Geometry: see drawing. Coordinates: mm, zero at the bounding-box minimum. A direction names the side the tool comes from. Coordinates: 2 decimals unless noted, no trailing zeros. Loops run counter-clockwise (first coordinate to the right, second up) from the corner with the lowest first, then second, coordinate; pieces in that order, holes last.
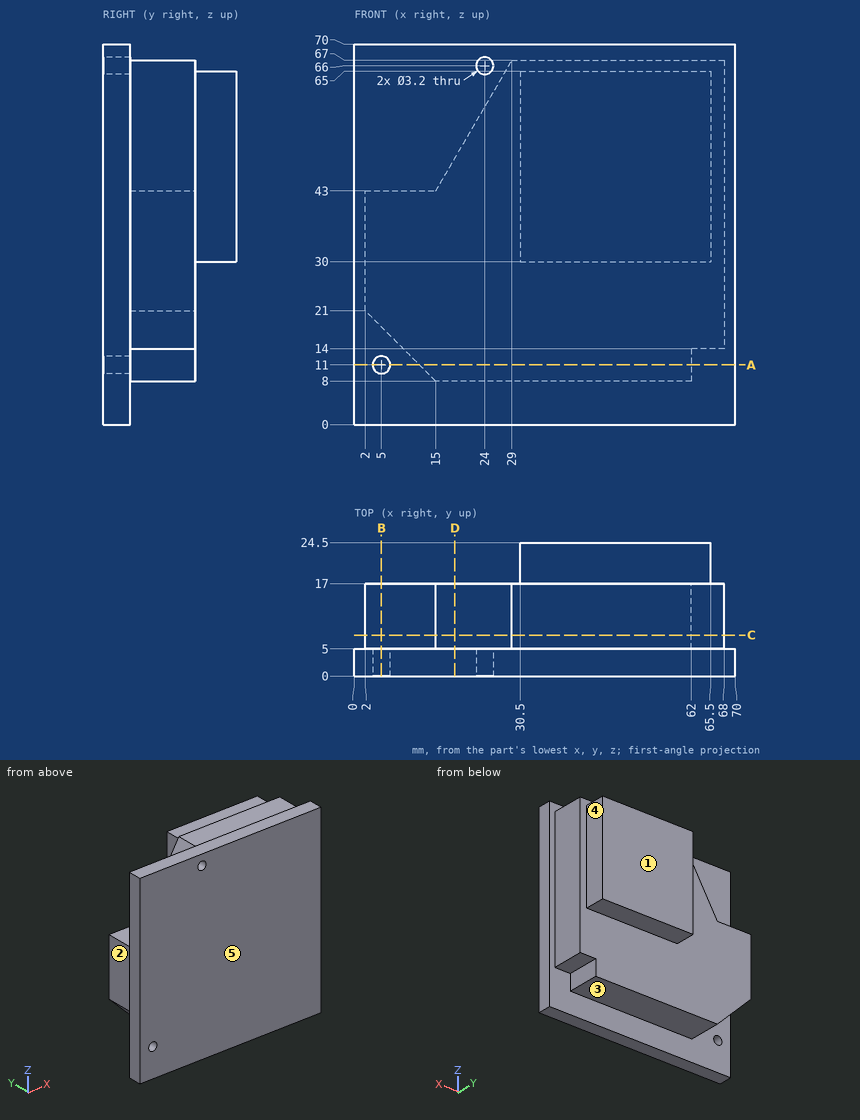
Item 1: Contact query for flat-ended pins moving along their axis: P1, Ø17.5, axis at x = 22.5, z = 31.5, coming from the +Y side; P2, Ø10, axis at x = 17, y = 20, coming from the +Z side; P3, Ø2.5, axis at x = 5, z = 11, coming from the -Y side; P4, Ø2, axis at x = 55.5, y = 18.5, coming from the -Z side. Output: stop coordinate, or through.
Result:
P1: stops at y = 24.5
P2: stops at z = 53.29
P3: passes through
P4: stops at z = 30
Item 2: Section query A-A (z = 11). Output: boundary loops of the cut face in (x, y).
Result:
outline: (0, 0) - (3.4, 0) - (3.4, 5) - (0, 5) - close; (6.6, 0) - (70, 0) - (70, 5) - (62, 5) - (62, 17) - (12, 17) - (12, 5) - (6.6, 5) - close
Item 3: Reachability of the marked faces 1, 2, 3, 4 and 5 from +Z, -Z, +X, -X, +Y, -Y: full face, straight path, thin tool, end or side. Return the list, or none.
Result:
face 1: +Z, -Z, +X, -X, +Y
face 2: +Z, -Z, -X, +Y
face 3: -Z, +X, -X, +Y
face 4: +Z, -Z, +X, +Y
face 5: +Z, -Z, +X, -X, -Y
Item 4: Section query C-C (y = 7.5). Output: boundary loops of the cut face in (x, z), then the cut area to 3 significant figures.
Result:
outline: (2, 21) - (15, 8) - (62, 8) - (62, 14) - (68, 14) - (68, 67) - (29, 67) - (15, 43) - (2, 43) - close
area: 3,290 mm2
Item 5: Line query: L1, parallel to Z at x = 5, y = 1.75; L2, parallel to Z at x = 24, y = 3.9; L3, parallel to X at y = 3.1, z = 66. Output: solid intervals per line, ascending.
Result:
L1: z = 0 to 9.4, 12.6 to 70
L2: z = 0 to 64.4, 67.6 to 70
L3: x = 0 to 22.4, 25.6 to 70
Item 6: Section query D-D (x = 18.5). Output: boundary loops of the cut face in (y, z).
Result:
outline: (0, 0) - (5, 0) - (5, 8) - (17, 8) - (17, 49) - (5, 49) - (5, 70) - (0, 70) - close
Item 7: Section query B-B (x = 5). Output: boundary loops of the cut face in (y, z).
Result:
outline: (0, 0) - (5, 0) - (5, 9.4) - (0, 9.4) - close; (0, 12.6) - (5, 12.6) - (5, 18) - (17, 18) - (17, 43) - (5, 43) - (5, 70) - (0, 70) - close
